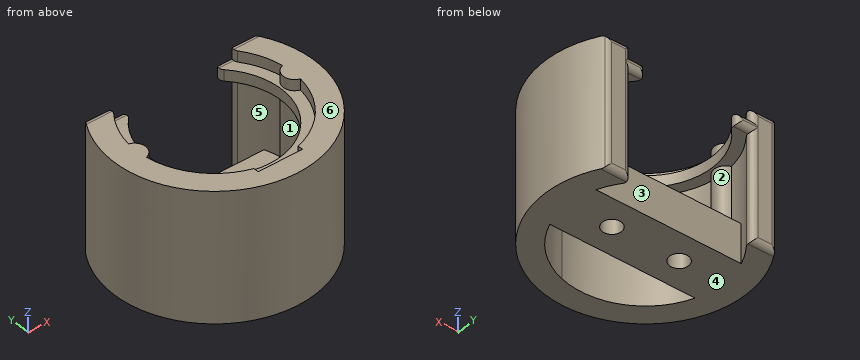
from build123d import *

# Parameters (mm, degrees)
SKETCH_3_R          = 6.95
SKETCH_3_R_2        = 5.95
EXTRUDE_3_DEPTH     = 1
SKETCH_1_R          = 8.95
EXTRUDE_1_DEPTH     = 11.6
CUT_EXTRUDE_1_DEPTH = 18.16872156
FILLET_4_R          = 0.5
SKETCH_5_W          = 17.187495454
SKETCH_5_H          = 5
EXTRUDE_4_DEPTH     = 3.5
SKETCH_6_W          = 0.98
SKETCH_6_H          = 0.456526807
CUT_EXTRUDE_2_DEPTH = 3.95
CUT_EXTRUDE_3_REACH = 19.169
SKETCH_8_R          = 0.85


with BuildPart() as part:
    # 草图3 → 凸台-拉伸3 (new body)
    with BuildSketch(Plane(origin=(0, 0, -0.98), x_dir=(-1, 0, 0), z_dir=(0, 0, -1))):
        with Locations(Location((0, 0, 0), (0, 0, 90))):
            Circle(SKETCH_3_R)
        with Locations(Location((0, 0, 0), (0, 0, 90))):
            Circle(SKETCH_3_R_2, mode=Mode.SUBTRACT)
    extrude(amount=EXTRUDE_3_DEPTH)

    # 草图1 → 凸台-拉伸1 (add)
    with BuildSketch(Plane.XY):
        Circle(SKETCH_1_R)
        with BuildLine():
            ThreePointArc((1.975, 6.663473193), (-3.760818846, 5.844548024), (-6.882867133, 0.963659707))
            ThreePointArc((-6.882867133, 0.963659707), (-6.15, 0), (-6.882867133, -0.963659707))
            ThreePointArc((-6.882867133, -0.963659707), (-3.760818846, -5.844548024), (1.975, -6.663473193))
            ThreePointArc((1.975, -6.663473193), (5.266632793, -4.53487365), (6.882867133, -0.963659707))
            ThreePointArc((6.882867133, -0.963659707), (6.15, 0), (6.882867133, 0.963659707))
            ThreePointArc((6.882867133, 0.963659707), (5.266632793, 4.53487365), (1.975, 6.663473193))
        make_face(mode=Mode.SUBTRACT)
    extrude(amount=-EXTRUDE_1_DEPTH)

    # 草图4 → 切除-拉伸1 (cut, through all)
    with BuildSketch(Plane.XY):
        with BuildLine():
            Line((-7.423105819, 5), (7.423105819, 5))
            ThreePointArc((7.423105819, 5), (0, 8.95), (-7.423105819, 5))
        make_face()
    extrude(amount=-CUT_EXTRUDE_1_DEPTH, mode=Mode.SUBTRACT)

    # 圆角4
    fillet_4_edges = [part.edges().sort_by_distance(p)[0] for p in [
        (6.125186063, 5, -11.6),
        (-6.125186063, 5, 0),
        (6.125186063, 5, 0),
        (4.827266307, 5, -0.49),
        (4.026278496, 5, -0.98),
        (4.827266307, 5, -6.79),
        (7.423105819, 5, -5.8),
        (-4.026278496, 5, -0.98),
        (-4.827266307, 5, -0.49),
        (-6.125186063, 5, -11.6),
        (-4.827266307, 5, -6.79),
        (-7.423105819, 5, -5.8),
        (-3.225290685, 5, -1.48),
        (-4.026278496, 5, -1.98),
        (4.026278496, 5, -1.98),
        (3.225290685, 5, -1.48),
    ]]
    fillet(fillet_4_edges, radius=FILLET_4_R - 0.0001)  # a hair under: the kernel refuses the full size

    # 草图5 → 凸台-拉伸4 (add)
    with BuildSketch(Plane(origin=(0, 0, -11.6), x_dir=(-1, 0, 0), z_dir=(0, 0, -1))):
        Rectangle(SKETCH_5_W, SKETCH_5_H)
    extrude(amount=-EXTRUDE_4_DEPTH)

    # 草图6 → 切除-拉伸2 (cut)
    with BuildSketch(Plane(origin=(1.975, 0, 0), x_dir=(0, 0, -1), z_dir=(1, 0, 0))):
        with Locations((0.49, -6.891736597)):
            Rectangle(SKETCH_6_W, SKETCH_6_H)
    extrude(amount=-CUT_EXTRUDE_2_DEPTH, mode=Mode.SUBTRACT)

    # 草图8 → 切除-拉伸3 (cut, up to next)
    with BuildSketch(Plane(origin=(0, 0, -11.6), x_dir=(-1, 0, 0), z_dir=(0, 0, -1)), mode=Mode.PRIVATE) as cut_extrude_3_sk1:
        with Locations((-3, 0)):
            Circle(SKETCH_8_R)
    cut_extrude_3_tool1 = extrude(cut_extrude_3_sk1.sketch, amount=-CUT_EXTRUDE_3_REACH, mode=Mode.PRIVATE) & part.part
    # 草图8 → 切除-拉伸3 (cut, up to next)
    with BuildSketch(Plane(origin=(0, 0, -11.6), x_dir=(-1, 0, 0), z_dir=(0, 0, -1)), mode=Mode.PRIVATE) as cut_extrude_3_sk2:
        with Locations((3, 0)):
            Circle(SKETCH_8_R)
    cut_extrude_3_tool2 = extrude(cut_extrude_3_sk2.sketch, amount=-CUT_EXTRUDE_3_REACH, mode=Mode.PRIVATE) & part.part
    add(cut_extrude_3_tool1.solids().sort_by_distance((3, 0, -11.6))[0], mode=Mode.SUBTRACT)
    add(cut_extrude_3_tool2.solids().sort_by_distance((-3, 0, -11.6))[0], mode=Mode.SUBTRACT)


solid = part.part
The model under review builds one solid part; all positions refer to its coordinate system, in mm. Face numbers are marked on the shaded views. A direction names the side the tool comes from. Coordinates: 2 decimals unless noted, no trailing zeros. Loops run counter-clockwise (first coordinate to the right, second up) from the corner with the lowest first, then second, coordinate; pieces in that order, holes last. Notation, with made-up numbers: (51, 86.5) -> (64, 86.5) arc R13 cw to (64, 106.5) -> close; hole circle Ø5 at (48.5, 79.5). An arc over 180 degrees is marked (long way). Use a Markdown table: item, result. Add a question column.
1. Add section B-B on x = 0. Write out the cut boundary in (y, z), plus the area to 3 significant figures.
2. Add section C-C on z = -3.5. Write out the cut boundary in (x, y) (3 decimals).
3. Add section A-A on y = 0. Write out the cut boundary in (x, z).
4. Add section D-D on x = 2.5. Write out the cut boundary in (y, z), plus the area to 3 significant figures.
5. Draft analysis for pull direction Z (two halves, no side actions). For the marked faces 1, 2, 3 and 4, state which applies: pulls with the +Z half, pulls with the -Z half, needs draft (parallel to the pull), parting line crosses it, or undercut.
6. To check wall thickness, follow line 1 (X direction, y = 0, z = -1.3); line 2 (X direction, y = 4.5, z = -3.75); line 3 (Y direction, x = -3, z = -10.1). State the ranges of each line that lie inside material, in increasing order.
7. Clearance check with flat-ended pins moving along their axes: pin 1 Ø1.5 at (x, y) = (3, 0) entering from -Z; pin 2 Ø5 at (x, y) = (2, -6) entering from +Z; pin 3 Ø1.5 at (x, y) = (3, -0.5) entering from +Z; pin 4 Ø6 at (x, y) = (1, -3.5) entering from +Z. State where each tip first meets the part, or that it passes through.
8. Machinability: for the marked faces 5 and 6, which of the approach directions +Z, -Z, +X, -X, +Y, -Y give a long, thin tool a straight path to every point of the face, cutting with its end or side? Answer none if there is none.
Returned:
| question | item | result |
|---|---|---|
| 1 | outline | (-8.95, -11.6) -> (-6.95, -11.6) -> (-6.95, -1.98) -> (-5.95, -1.98) -> (-5.95, -0.98) -> (-7.12, -0.98) -> (-7.12, 0) -> (-8.95, 0) -> close; (-2.5, -11.6) -> (2.5, -11.6) -> (2.5, -8.1) -> (-2.5, -8.1) -> close |
| 1 | area | 41.5 mm² |
| 2 | outline | (-7.575, 4.766) arc R8.95 ccw (long way) to (7.575, 4.766) arc R0.5 ccw to (7.152, 5) -> (5.937, 5) arc R0.5 ccw to (5.539, 4.198) arc R6.95 cw to (6.883, 0.964) arc R1 ccw to (6.883, -0.964) arc R6.95 cw to (-6.883, -0.964) arc R1 ccw to (-6.883, 0.964) arc R6.95 cw to (-5.539, 4.198) arc R0.5 ccw to (-5.937, 5) -> (-7.152, 5) arc R0.5 ccw to start |
| 3 | outline | (-8.95, -11.6) -> (-3.85, -11.6) -> (-3.85, -8.1) -> (-6.15, -8.1) -> (-6.15, -1.98) -> (-5.95, -1.98) -> (-5.95, -0.98) -> (-6.15, -0.98) -> (-6.15, 0) -> (-8.95, 0) -> close; (-2.15, -11.6) -> (2.15, -11.6) -> (2.15, -8.1) -> (-2.15, -8.1) -> close; (3.85, -11.6) -> (8.95, -11.6) -> (8.95, 0) -> (6.15, 0) -> (6.15, -0.98) -> (5.95, -0.98) -> (5.95, -1.98) -> (6.15, -1.98) -> (6.15, -8.1) -> (3.85, -8.1) -> close |
| 4 | outline | (-8.59, -11.6) -> (-6.48, -11.6) -> (-6.48, -1.98) -> (-5.4, -1.98) -> (-5.4, -0.98) -> (-6.48, -0.98) -> (-6.48, 0) -> (-8.59, 0) -> close; (-2.5, -11.6) -> (-0.69, -11.6) -> (-0.69, -8.1) -> (-2.5, -8.1) -> close; (0.69, -11.6) -> (2.5, -11.6) -> (2.5, -8.1) -> (0.69, -8.1) -> close |
| 4 | area | 38.2 mm² |
| 5 | face 1 | undercut |
| 5 | face 2 | undercut |
| 5 | face 3 | needs draft |
| 5 | face 4 | pulls with the -Z half |
| 6 | line 1 | x = -8.95 to -5.95, 5.95 to 8.95 |
| 6 | line 2 | x = -7.74 to -5.44, 5.44 to 7.74 |
| 6 | line 3 | y = -8.43 to -6.27, -2.5 to -0.85, 0.85 to 2.5 |
| 7 | pin 1 | passes through |
| 7 | pin 2 | stops at z = 0 |
| 7 | pin 3 | stops at z = -8.1 |
| 7 | pin 4 | stops at z = -0.98 |
| 8 | face 5 | none |
| 8 | face 6 | +Z, +X, -X, +Y, -Y |
